Build history of the part. All positions in model axes, mm. Give positions to 0.01 mm unless a question says otherwise; leave off trailing zeros. Order: outer loops, then holes, each group sorted by start corner. A loop starts at its lowest first (then second) coordinate and runs counter-clockwise, first axis right, second up. Notation, with made-up numbers: (88, 54.5) -> (114, 54.5) arc R22 cw to (114, 91.5) -> close; hole circle Ø8 at (7.5, -34.75). An arc over 180 degrees is marked (long way). One line per item, written item: value. Start each with the question number.
(1) Saw through at A-A on y = 6.35. Give the cut face in (x, z) (3 decimals), plus the area to 3 significant figures.
(2) Saw through at B-B on x = 50.8. Give the cut face in (y, z) (3 decimals).
(3) Probe line 1 (Y direction, x = 50.8, z = -22) (3 decimals); line 2 (X direction, y = 5.25, z = 49.5); line 3 (X direction, y = 8, z = 24). List the from-to ranges inside material, lowest first.
(4) Saw through at D-D on x = -2.5. Give the cut face in (y, z), plus the area to 3 significant figures.
(5) Saw through at C-C on z = 3.5. Give the cut face in (x, y) (3 decimals).
(6) Two-plate mould, pull along X, no slides. Class faces 1 (the flat face through (-63.5, 6, 1)), 2 (the flat face through (27, 12.7, -1)), 3 (the cylindrical face through (16.426, 9.526, 0.889)): +X half, -X half, draft (parallel to the pull), parting line (faces both ways), or undercut.
(7) Pin check, flat tips, straight feed: pin 1 (3 mm diameter, centred on x = -4.5, z = 11.5, fed in from +Y); pin 2 (3 mm diameter, centred on x = 50.8, y = 6.35, fed in from -Z). Stop position of each tip, or through.
```python
from build123d import *

# Parameters (mm, degrees)
SKETCH2_W           = 127
SKETCH2_H           = 127
BOSS_EXTRUDE1_DEPTH = 12.7
FILLET1_R           = 7.62
SKETCH3_R           = 5.08
CUT_EXTRUDE1_DEPTH  = 143.557146436
LPATTERN1_COUNT     = 5
LPATTERN1_PITCH     = 21.59
SKETCH3_3_R         = 1.905
SKETCH3_3_R_2       = 5.08
CUT_EXTRUDE2_DEPTH  = 143.557146436


with BuildPart() as part:
    # Sketch2 → Boss-Extrude1 (new body)
    with BuildSketch(Plane(origin=(0, 0, 0), x_dir=(1, 0, 0), z_dir=(0, 1, 0))):
        Rectangle(SKETCH2_W, SKETCH2_H)
    extrude(amount=BOSS_EXTRUDE1_DEPTH)

    # Fillet1
    fillet1_edges = [part.edges().sort_by_distance(p)[0] for p in [
        (63.5, 6.35, 63.5),
        (-63.5, 6.35, 63.5),
        (-63.5, 6.35, -63.5),
        (63.5, 6.35, -63.5),
    ]]
    fillet(fillet1_edges, radius=FILLET1_R)

    # Sketch3 → Cut-Extrude1 (cut, through all)
    with BuildSketch(Plane.XY.offset(63.5)):
        with Locations((38.1, 14.605)):
            Circle(SKETCH3_R)
    cut_extrude1 = extrude(amount=-CUT_EXTRUDE1_DEPTH, mode=Mode.SUBTRACT)

    # LPattern1: Cut-Extrude1 ×5
    with Locations(*[(-i * LPATTERN1_PITCH, 0, 0) for i in range(1, LPATTERN1_COUNT)]):
        add(cut_extrude1, mode=Mode.SUBTRACT)

    # Sketch3<3> → Cut-Extrude2 (cut, through all)
    with BuildSketch(Plane.XY.offset(63.5)):
        with Locations((50.8, 6.35)):
            Circle(SKETCH3_3_R)
        with Locations((38.1, 14.605)):
            Circle(SKETCH3_3_R_2)
    extrude(amount=-CUT_EXTRUDE2_DEPTH, mode=Mode.SUBTRACT)


solid = part.part
```
Results below:
1. outline: (-63.5, -55.88) arc R7.62 ccw to (-55.88, -63.5) -> (48.895, -63.5) -> (48.895, 63.5) -> (-55.88, 63.5) arc R7.62 ccw to (-63.5, 55.88) -> close; (52.705, -63.5) -> (55.88, -63.5) arc R7.62 ccw to (63.5, -55.88) -> (63.5, 55.88) arc R7.62 ccw to (55.88, 63.5) -> (52.705, 63.5) -> close
1. area: 15,600 mm²
2. outline: (0, -63.5) -> (4.445, -63.5) -> (4.445, 63.5) -> (0, 63.5) -> close; (8.255, -63.5) -> (12.7, -63.5) -> (12.7, 63.5) -> (8.255, 63.5) -> close
3. line 1: y = 0 to 4.445, 8.255 to 12.7
3. line 2: x = -63.5 to 49.24, 52.36 to 63.5
3. line 3: x = -63.5 to 49.85, 51.75 to 63.5
4. outline: (0, -63.5) -> (10.23, -63.5) -> (10.23, 63.5) -> (0, 63.5) -> close
4. area: 1,300 mm²
5. outline: (-63.5, 0) -> (63.5, 0) -> (63.5, 12.7) -> (42.809, 12.7) arc R5.08 cw to (33.391, 12.7) -> (21.219, 12.7) arc R5.08 cw to (11.801, 12.7) -> (-0.371, 12.7) arc R5.08 cw to (-9.789, 12.7) -> (-21.961, 12.7) arc R5.08 cw to (-31.379, 12.7) -> (-43.551, 12.7) arc R5.08 cw to (-52.969, 12.7) -> (-63.5, 12.7) -> close; hole circle Ø3.81 at (50.8, 6.35)
6. face 1: -X half
6. face 2: draft
6. face 3: undercut
7. pin 1: stops at y = 9.97
7. pin 2: passes through
